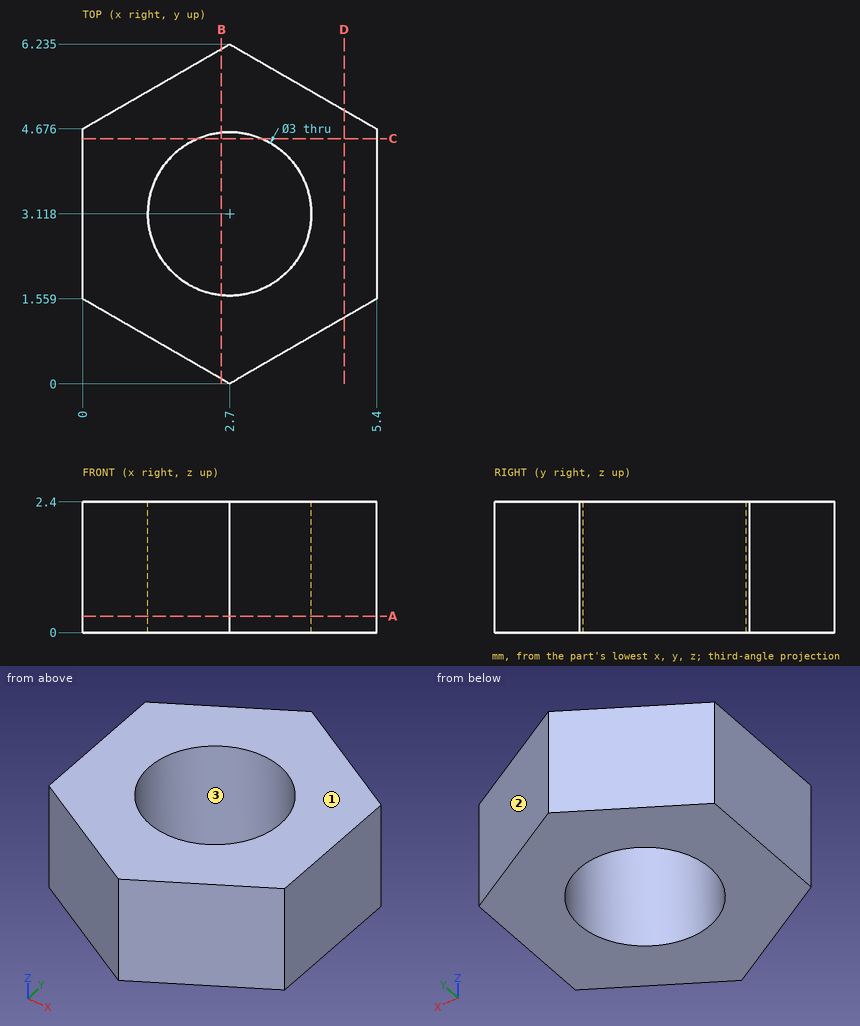
Geometry: see drawing. Coordinates: mm, zero at the bounding-box minimum. Give positions to 0.01 mm unless a question says otherwise; leave off trailing zeros. Loops run counter-clockwise (first coordinate to the right, second up) from the corner with the lowest first, then second, coordinate; pieces in that order, holes last. Notation, with made-up numbers: M 53.5,87.25 L 77.5,87.25 A10 ccw 77.5,91.25 Z; hole C 65,81.25 d7. An arc over 180 degrees is marked long. Answer as CSV lines item,"result". Start each with the question number.
1. Section C-C on y = 4.5. Return loops of the section in (x, z).
2. Pull-direction query (X, two-part tool) for the marked faces 1, 2 and 3; classes: released by +X, released by -X, zero draft, split by the parting line, or undercut.
3. Section B-B on x = 2.55. Return loops of the section in (y, z) (1 decimal).
4. Section D-D on x = 4.8. Return loops of the section in (y, z).
5. Section A-A on z = 0.3. Return loops of the section in (x, y) (1 decimal).
6. Line query: L1, parallel to X at y = 3.75, z = 0.7; L2, parallel to X at y = 3.25, z = 2.1 (1 decimal); L3, parallel to Y at x = 2.05, z = 1.35 (1 decimal). Output: solid intervals per line, ascending.
Computed values:
1,outline,"M 0,0 L 2.12,0 L 2.12,2.4 L 0,2.4 Z; M 3.28,0 L 5.4,0 L 5.4,2.4 L 3.28,2.4 Z"
2,face 1,"zero draft"
2,face 2,"released by +X"
2,face 3,"undercut"
3,outline,"M 0.1,0 L 1.6,0 L 1.6,2.4 L 0.1,2.4 Z; M 4.6,0 L 6.1,0 L 6.1,2.4 L 4.6,2.4 Z"
4,outline,"M 1.21,0 L 5.02,0 L 5.02,2.4 L 1.21,2.4 Z"
5,outline,"M 0,1.6 L 2.7,0 L 5.4,1.6 L 5.4,4.7 L 2.7,6.2 L 0,4.7 Z; hole C 2.7,3.1 d3"
6,L1,"x = 0 to 1.34, 4.06 to 5.4"
6,L2,"x = 0 to 1.2, 4.2 to 5.4"
6,L3,"y = 0.4 to 1.8, 4.5 to 5.9"
